Geometry: final body of the model. Coordinates: model frame, mm. A direction names the side the tool comes from. Give positions to 0.01 mm unless a question says otherwise; leave off trailing zeros. Loops run counter-clockwise (first coordinate to the right, second up) from the corner with the lowest first, then second, coordinate; pieces in that order, holes last. Notation, with made-up numbers: M -8,-10 L 31,-10 A13 cw 31,7 Z; hole C 3,13.5 d3. An arc over 180 degrees is marked long. One line per question, with ' | ' between items. Start each with the question number.
from build123d import *

# Parameters (mm, degrees)
SKETCH1_R           = 36.83
BOSS_EXTRUDE1_DEPTH = 63.5
SKETCH4_W           = 73.66
SKETCH4_H           = 114.3
BOSS_EXTRUDE2_DEPTH = 63.5
SKETCH5_W           = 73.66
SKETCH5_H           = 73.66
BOSS_EXTRUDE3_DEPTH = 76.2
SKETCH6_R           = 12.7
BOSS_EXTRUDE4_DEPTH = 50.8
SKETCH2_R           = 13.97
CUT_EXTRUDE1_DEPTH  = 48.26


with BuildPart() as part:
    # Sketch1 → Boss-Extrude1 (new body)
    with BuildSketch(Plane.XY):
        Circle(SKETCH1_R)
    extrude(amount=BOSS_EXTRUDE1_DEPTH)

    # Sketch4 → Boss-Extrude2 (add, through all)
    with BuildSketch(Plane.XY):
        with Locations((0, 57.15)):
            Rectangle(SKETCH4_W, SKETCH4_H)
    extrude(amount=BOSS_EXTRUDE2_DEPTH)

    # Sketch5 → Boss-Extrude3 (add)
    with BuildSketch(Plane.XY):
        with Locations((0, 77.47)):
            Rectangle(SKETCH5_W, SKETCH5_H)
    extrude(amount=-BOSS_EXTRUDE3_DEPTH)

    # Sketch6 → Boss-Extrude4 (add)
    with BuildSketch(Plane.ZY.offset(36.83)):
        with Locations(Location((-6.35, 76.2, 0), (0, 0, 90))):
            Circle(SKETCH6_R)
    extrude(amount=BOSS_EXTRUDE4_DEPTH)

    # Sketch2 → Cut-Extrude1 (cut)
    with BuildSketch(Plane.XY):
        with Locations(Location((0, 0, 0), (0, 0, 180))):
            Circle(SKETCH2_R)
    extrude(amount=CUT_EXTRUDE1_DEPTH, mode=Mode.SUBTRACT)


solid = part.part
Q1. Section C-C, the plane x = -8.5. Output: boundary loops of the cut face in (y, z), plus the area to 3 significant figures.
Q2. Section B-B, the plane y = 76.2. Output: boundary loops of the cut face in (x, z), plus the area to 3 significant figures.
Q3. Section A-A, the plane z = 37.5. Output: boundary loops of the cut face in (x, y), plus the area to 3 significant figures.
Q4. Set-up query: faces 5 (the flat face through (0, 0, 48.26)), 6 (the flat face through (-9, 11, 0)), 7 (the flat face through (-1, 78, -76.2)). Return all of +Z, -Z, +X, -X, +Y, -Y with unobstructed straight access to the full face (end or side cutting, diameter ignored); none if empty.
Q5. Material intervals for L1, parallel to Y at x = 0, z = 24; L2, parallel to Y at x = -9.5, z = -33; L3, parallel to Z at x = 26, y = 5, sorted ascending.
Q6. Contact query for flat-ended pins moving along their axis: pin 1 (1.5 mm diameter, centred on y = -21.5, z = 26.5, fed in from +X); pin 2 (4 mm diameter, centred on x = -10.5, z = -58, fed in from -Y); pin 3 (22 mm diameter, centred on x = 14.5, y = -8, fed in from -Z). Output: stop coordinate, or through.
Q7. Section D-D, the plane z = -24.5. Output: boundary loops of the cut face in (x, y).
Q8. Draft query along Y for faces 1 (the cylindrical face through (1.82, -13.85, 23.79)), 2 (the cylindrical face through (-61.874, 63.512, -6.908)), 3 (the flat face through (-1, 114.3, -5)), 4 (the flat face through (-87.63, 76, -7)). Return one class per face: released by +Y, released by -Y, zero draft, split by the parting line, or undercut.
Model answer:
1) outline: M -35.84,0 L -11.09,0 L -11.09,48.26 L 11.09,48.26 L 11.09,0 L 40.64,0 L 40.64,-76.2 L 114.3,-76.2 L 114.3,63.5 L -35.84,63.5 Z | area: 14,100 mm^2
2) outline: M -87.63,-19.05 L -36.83,-19.05 L -36.83,-76.2 L 36.83,-76.2 L 36.83,63.5 L -36.83,63.5 L -36.83,6.35 L -87.63,6.35 Z | area: 11,600 mm^2
3) outline: M -36.83,0 A36.83 ccw 36.83,0 L 36.83,114.3 L -36.83,114.3 Z; hole C 0,0 d27.94 | area: 9,940 mm^2
4) face 5: -Z | face 6: -Z, +X, -X, -Y | face 7: -Z, +X, -X, +Y, -Y
5) L1: y = -36.83 to -13.97, 13.97 to 114.3 | L2: y = 40.64 to 114.3 | L3: z = 0 to 63.5
6) pin 1: stops at x = 30.43 | pin 2: stops at y = 40.64 | pin 3: stops at z = 0
7) outline: M -36.83,40.64 L 36.83,40.64 L 36.83,114.3 L -36.83,114.3 Z
8) face 1: undercut | face 2: split by the parting line | face 3: released by +Y | face 4: zero draft
